from build123d import *

# Parameters (mm, degrees)
F1_DEPTH = 32
F2_SIZE  = 5
F3_SIZE  = 5
F4_R     = 6.5
F5_DEPTH = 88.001
F6_R     = 5.5
F7_DEPTH = 13.001


with BuildPart() as f1:
    # F0 (on Front) → F1 (new body)
    with BuildSketch(Plane.XZ):
        Polygon((0, 13), (0, 0), (39, 0), (39, 17), (74, 17), (74, 0), (113, 0), (113, 13), (88, 13), (88, 64), (69, 64), (69, 30), (44, 30), (44, 64), (25, 64), (25, 13), align=None)
    extrude(amount=F1_DEPTH)

    # F2
    f2_edges = [f1.edges().sort_by_distance(p)[0] for p in [
        (113, -32, 6.5),
    ]]
    chamfer(f2_edges, length=F2_SIZE)

    # F3
    f3_edges = [f1.edges().sort_by_distance(p)[0] for p in [
        (0, -32, 6.5),
    ]]
    chamfer(f3_edges, length=F3_SIZE)

    # F4 (on face) → F5 (cut, through all)
    with BuildSketch(Plane.YZ.offset(88)):
        with Locations((-16, 46)):
            Circle(F4_R)
    extrude(amount=-F5_DEPTH, mode=Mode.SUBTRACT)

    # F6 (on face) → F7 (cut, through all)
    with BuildSketch(Plane.XY.offset(13)):
        with Locations((13, -13)):
            Circle(F6_R)
        with Locations((100, -13)):
            Circle(F6_R)
    extrude(amount=-F7_DEPTH, mode=Mode.SUBTRACT)


solid = f1.part
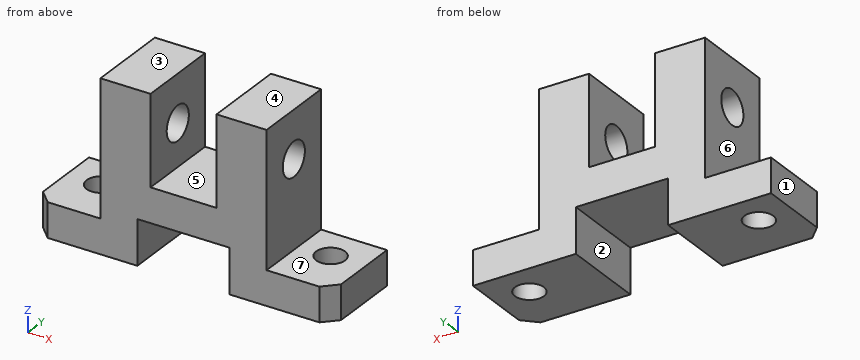
Input: part model. Units: mm. Frame: model coordinates. Face numbers are marked on the shaded views. A direction names the side the tool comes from. Coordinates: 2 decimals unless noted, no trailing zeros. Order: outer loops, then holes, each group sorted by start corner. A loop starts at its lowest first (then second) coordinate and runs counter-clockwise, first axis right, second up. Notation, with made-up numbers: M -25.5,58 L -10.5,58 A6 ccw -10.5,64 Z; hole C 0,9.25 d8. An arc over 180 degrees is marked long. Answer in a Markdown table with one row per item.
(1) Section query B-B, the plane x = 13. Output: boundary loops of the cut face in (y, z), plus the area to 3 significant figures.
Numbers:
| item | result |
|---|---|
| outline | M -32,0 L -18.5,0 L -18.5,13 L -32,13 Z; M -7.5,0 L 0,0 L 0,13 L -7.5,13 Z |
| area | 273 mm^2 |
(2) Access query for the marked faces 4, 5, 6 and 7. Directions: +Z, -Z, +X, -X, +Y, -Y. A direction counts if a zero-diameter tool reaches every point of the face in a straight line with its end or side. Return the directions, or none.
Numbers:
| item | result |
|---|---|
| face 4 | +Z, +X, -X, +Y, -Y |
| face 5 | +Z, +Y, -Y |
| face 6 | +Z, -X, +Y, -Y |
| face 7 | +Z, +X, +Y, -Y |
(3) Section query C-C, the plane z = 46. Output: boundary loops of the cut face in (x, y).
Numbers:
| item | result |
|---|---|
| outline | M 25,-32 L 44,-32 L 44,-22.5 L 25,-22.5 Z; M 25,-9.5 L 44,-9.5 L 44,0 L 25,0 Z; M 69,-32 L 88,-32 L 88,-22.5 L 69,-22.5 Z; M 69,-9.5 L 88,-9.5 L 88,0 L 69,0 Z |
(4) Draft query along X for the marked faces 1, 2 and 3. Return one class per face: pulls with the +X half, pulls with the -X half, needs draft (parallel to the pull), parting line crosses it, or undercut.
Numbers:
| item | result |
|---|---|
| face 1 | pulls with the -X half |
| face 2 | undercut |
| face 3 | needs draft |
(5) Material intervals for line 1 (Z direction, x = 31, y = -16); line 2 (Z direction, x = 39.75, y = -16); line 3 (X direction, y = -18.5, z = 56), sorted ascending. Write a range as [from, to].
Numbers:
| item | result |
|---|---|
| line 1 | z = [0, 39.5], [52.5, 64] |
| line 2 | z = [17, 39.5], [52.5, 64] |
| line 3 | x = [25, 44], [69, 88] |
(6) Section query A-A, the plane z = 6.5. Output: boundary loops of the cut face in (x, y), plus the area to 3 significant figures.
Numbers:
| item | result |
|---|---|
| outline | M 0,-27 L 5,-32 L 39,-32 L 39,0 L 0,0 Z; M 74,-32 L 108,-32 L 113,-27 L 113,0 L 74,0 Z; hole C 13,-13 d11; hole C 100,-13 d11 |
| area | 2,280 mm^2 |
(7) Section query D-D, the plane x = 37. Output: boundary loops of the cut face in (y, z), plus the area to 3 significant figures.
Numbers:
| item | result |
|---|---|
| outline | M -32,0 L 0,0 L 0,64 L -32,64 Z; hole C -16,46 d13 |
| area | 1,920 mm^2 |
(8) Contact query for flat-ended pins moving along their axis: pin 1 Ø1 at (y, z) = (-8, 47.5) entering from +X; pin 2 Ø15 at (y, z) = (-16, 46) entering from -X; pin 3 Ø12.5 at (x, y) = (102.5, -13) entering from +Z; pin 4 Ø1.5 at (x, y) = (78, -25) entering from -Z. Output: stop coordinate, or through.
Numbers:
| item | result |
|---|---|
| pin 1 | stops at x = 88 |
| pin 2 | stops at x = 25 |
| pin 3 | stops at z = 13 |
| pin 4 | stops at z = 0 |
